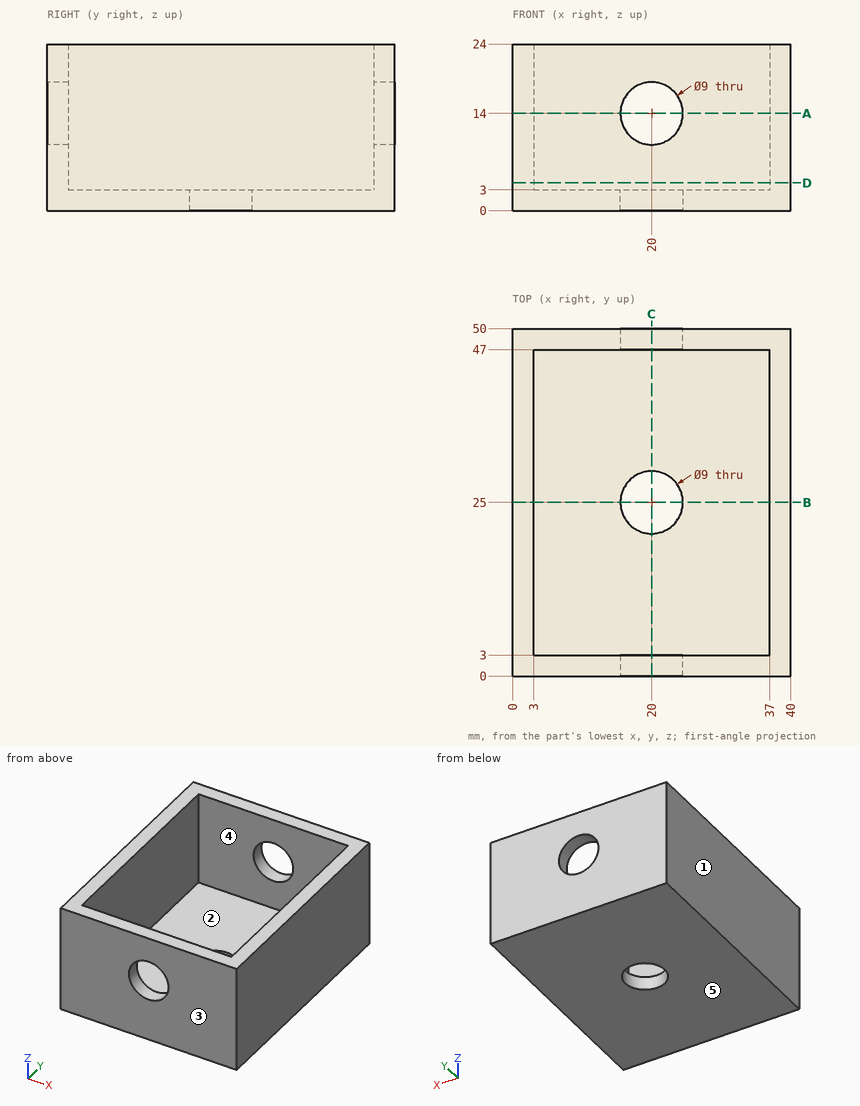
Verification items for this drawing (mm, ordinates from the low corner). A direction names the side the tool comes from. Coordinates: 2 decimals unless noted, no trailing zeros. Loops run counter-clockwise (first coordinate to the right, second up) from the corner with the lowest first, then second, coordinate; pieces in that order, holes last. Notation, with made-up numbers: (55.25, 7) - (83.25, 7) arc R20 ccw to (83.25, 35) - close; hole circle Ø2 at (43.5, 30.5). An arc over 180 degrees is marked (long way). Use one line per item in the form item = value. Start each with the question number.
Item 1: Section check C-C, the plane x = 20. Enter the section's corners in (y, z).
Item 2: Tool access check on the marked faces 1 and 2. Record the directions out of +Z, -Z, +X, -X, +Y, -Y that give a thin tool (end or side, any length) a straight path to the whole face; none if there is none.
Item 3: Section check B-B, the plane y = 25. Enter the section's corners in (x, z).
Item 4: Section check D-D, the plane z = 4. Enter the section's corners in (x, y), and give its area (3 significant figures).
Item 5: Section check A-A, the plane z = 14. Enter the section's corners in (x, y).
Item 6: Mould release check, pull along Y, two halves, no side actions. Record for the marked faces 3, 4 and 5: +Y half, -Y half, draft (parallel to the pull), parting line (faces both ways), or undercut.
Item 7: Thickness scan on probe 1 along Y at (x, z) = (23.5, 10.75); probe 2 along X at (y, z) = (37.5, 16.25); probe 3 along Y at (x, z) = (20, 2.2). Record the ranges inside material, lowest first.
Item 8: Gauge pin test, flat ends, axial feed: pin 1 (2 mm diameter, centred on x = 22.5, z = 16.5, fed in from -Y); pin 2 (10.5 mm diameter, centred on x = 20, y = 25, fed in from +Z). Record the tip position at first contact, or that the pin passes through.
Computed:
q1.outline = (0, 0) - (20.5, 0) - (20.5, 3) - (3, 3) - (3, 9.5) - (0, 9.5) - close; (0, 18.5) - (3, 18.5) - (3, 24) - (0, 24) - close; (29.5, 0) - (50, 0) - (50, 9.5) - (47, 9.5) - (47, 3) - (29.5, 3) - close; (47, 18.5) - (50, 18.5) - (50, 24) - (47, 24) - close
q2.face_1 = +Z, -Z, -X, +Y, -Y
q2.face_2 = +Z
q3.outline = (0, 0) - (15.5, 0) - (15.5, 3) - (3, 3) - (3, 24) - (0, 24) - close; (24.5, 0) - (40, 0) - (40, 24) - (37, 24) - (37, 3) - (24.5, 3) - close
q4.outline = (0, 0) - (40, 0) - (40, 50) - (0, 50) - close; hole (3, 3) - (37, 3) - (37, 47) - (3, 47) - close
q4.area = 504 mm2
q5.outline = (0, 0) - (15.5, 0) - (15.5, 3) - (3, 3) - (3, 47) - (15.5, 47) - (15.5, 50) - (0, 50) - close; (24.5, 0) - (40, 0) - (40, 50) - (24.5, 50) - (24.5, 47) - (37, 47) - (37, 3) - (24.5, 3) - close
q6.face_3 = -Y half
q6.face_4 = undercut
q6.face_5 = draft
q7.probe_1 = 0 to 3, 47 to 50
q7.probe_2 = 0 to 3, 37 to 40
q7.probe_3 = 0 to 20.5, 29.5 to 50
q8.pin_1 = 0
q8.pin_2 = 3
